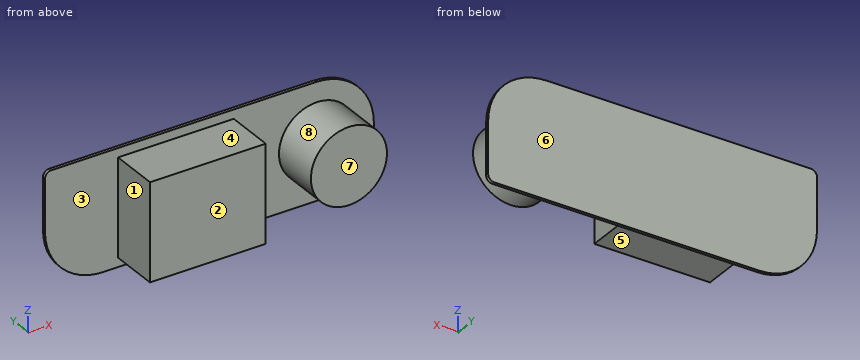
from build123d import *

# Parameters (mm, degrees)
F1_DEPTH = 1
F2_W     = 38
F2_H     = 32
F2_R     = 12.5
F3_DEPTH = 16


with BuildPart() as f1:
    # F0 (on Front) → F1 (new body)
    with BuildSketch(Plane.XZ):
        with BuildLine():
            ThreePointArc((54, 0), (48.435029, 13.435029), (35, 19))
            Line((35, 19), (-52, 19))
            ThreePointArc((-52, 19), (-53.414214, 18.414214), (-54, 17))
            Line((-54, 17), (-54, 0))
            ThreePointArc((-54, 0), (-48.435029, -13.435029), (-35, -19))
            Line((-35, -19), (52, -19))
            ThreePointArc((52, -19), (53.414214, -18.414214), (54, -17))
            Line((54, -17), (54, 0))
        make_face()
    extrude(amount=F1_DEPTH)

    # F2 (on face) → F3 (join)
    with BuildSketch(Plane.XZ.offset(1)):
        with Locations((-11, 0)):
            Rectangle(F2_W, F2_H)
        with Locations((35.345, 0)):
            Circle(F2_R)
    extrude(amount=F3_DEPTH)


solid = f1.part
Build history of the part. All positions in model axes, mm. Face numbers are marked on the shaded views. A direction names the side the tool comes from. Round coordinates to 2 decimals unless told otherwise and drop trailing zeros. Write each loop counter-clockwise with the first axis right and the second up, starting at its lowest first coordinate (ties: lowest second). Pieces come first, ordered by that corner, then holes. Notation, with made-up numbers: M -33.75,-20.75 L -13.75,-20.75 A21 cw -13.75,-2.75 Z; hole C 21,-9.75 d6. An arc over 180 degrees is marked long. Answer as a JSON object with one key per item and string values. Group by question number.
(1) Cut at A-A (y = -12.75). Give the cut face in (x, z) (3 decimals), and give its area (3 significant figures).
(2) Drill centre lines: L1, parallel to Y at x = -38, z = -3; L2, parallel to Z at x = -29, y = -11.75; L3, parallel to X at y = -2, z = -6.5. Where is each one in solid material? Low to high.
(3) Mould opens along X. For the marked faces 1, 2 and 3 say: pulls with the +X half, pulls with the -X half, needs draft (parallel to the pull), parting line crosses it, or undercut.
(4) Cut at B-B (x = -13). Give the cut face in (y, z).
(5) Flat gauge pins, fed straight in: pin 1 (1 mm diameter, centred on x = -8, y = -2.5, fed in from -Z); pin 2 (2 mm diameter, centred on y = -7, z = -14.5, fed in from +X); pin 3 (5 mm diameter, centred on y = -8, z = -3.5, fed in from -X). Where does each tip first touch, or does it go through?
(6) Which spindle directions (+Z, -Z, +X, -X, +Y, -Y) get a long thin tool onto all of the face, cutting with end or side? Do the marked faces 4, 5, 6, 7 and 8. Say none if no direction does.
(7) Cut at C-C (z = 6.5). Give the cut face in (x, y), and give its area (3 significant figures).
(8) Cut at D-D (z = 15). Give the cut face in (x, y), and give its area (3 significant figures).
Responses:
{
 "1": {"outline": "M -30,-16 L 8,-16 L 8,16 L -30,16 Z; C 35.345,0 d25", "area": "1,710 mm2"},
 "2": {"L1": "y = -1 to 0", "L2": "z = -16 to 16", "L3": "x = -30 to 8, 24.67 to 46.02"},
 "3": {"face 1": "pulls with the -X half", "face 2": "needs draft", "face 3": "undercut"},
 "4": {"outline": "M -17,-16 L -1,-16 L -1,-19 L 0,-19 L 0,19 L -1,19 L -1,16 L -17,16 Z"},
 "5": {"pin 1": "stops at z = -16", "pin 2": "stops at x = 8", "pin 3": "stops at x = -30"},
 "6": {"face 4": "+Z, +X, -X, -Y", "face 5": "-Z, +X, -X, -Y", "face 6": "+Z, -Z, +X, -X, +Y", "face 7": "+Z, -Z, +X, -X, -Y", "face 8": "-Y"},
 "7": {"outline": "M -54,-1 L -30,-1 L -30,-17 L 8,-17 L 8,-1 L 24.67,-1 L 24.67,-17 L 46.02,-17 L 46.02,-1 L 52.85,-1 L 52.85,0 L -54,0 Z", "area": "1,060 mm2"},
 "8": {"outline": "M -54,-1 L -30,-1 L -30,-17 L 8,-17 L 8,-1 L 46.66,-1 L 46.66,0 L -54,0 Z", "area": "709 mm2"}
}
